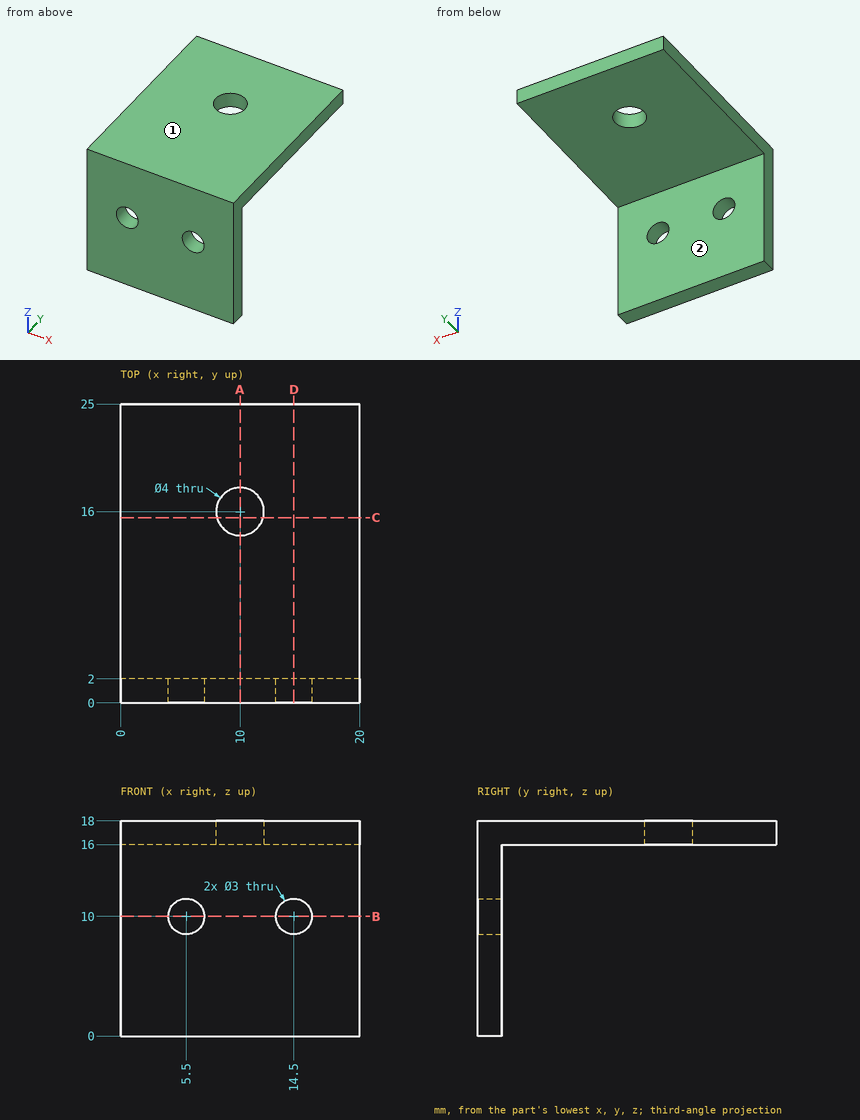
Input: dimensioned drawing with shaded views. Units: mm. Origin: part minimum x, y, z. A direction names the side the tool comes from. Coordinates: 2 decimals unless noted, no trailing zeros. Order: outer loops, then holes, each group sorted by start corner. A loop starts at its lowest first (then second) coordinate and runs counter-clockwise, first axis right, second up. Notation, with made-up numbers: (3, 28) - (59, 28) arc R31 ccw to (59, 54) - close; hole circle Ø4 at (58, 61.25). An arc over 180 degrees is marked (long way). Return JSON: item names as keys, results as strings. Group by question number.
1. Pin query (flat end, axial travel): pin 1 (6 mm diameter, centred on x = 8.5, y = 15.5, fed in from -Z); pin 2 (3.5 mm diameter, centred on x = 14.5, z = 10, fed in from +Y). Return the tip coordinate at first contact, or that it passes through.
2. Material intervals for line 1 along X through (y, z) = (1.1, 10); line 2 along Y through (x, z) = (10, 17.4); line 3 along Z through (x, y) = (14.5, 1.4), sorted ascending. Write a range as [from, to].
3. Cut plane A-A (x = 10). Output: boundary loops of the cut face in (y, z), plus the area to 3 significant figures.
4. Cut plane D-D (x = 14.5). Output: boundary loops of the cut face in (y, z).
5. Cut plane B-B (z = 10). Output: boundary loops of the cut face in (x, y).
6. Cut plane C-C (y = 15.5). Output: boundary loops of the cut face in (x, z), plus the area to 3 significant figures.
7. Set-up query: the marked faces 1 and 2. Return all of +Z, -Z, +X, -X, +Y, -Y with unobstructed straight access to the full face (end or side cutting, diameter ignored); none if empty.
Resolved:
{
 "1": {"pin 1": "stops at z = 16", "pin 2": "stops at y = 2"},
 "2": {"line 1": "x = [0, 4], [7, 13], [16, 20]", "line 2": "y = [0, 14], [18, 25]", "line 3": "z = [0, 8.5], [11.5, 18]"},
 "3": {"outline": "(0, 0) - (2, 0) - (2, 16) - (14, 16) - (14, 18) - (0, 18) - close; (18, 16) - (25, 16) - (25, 18) - (18, 18) - close", "area": "74.0 mm²"},
 "4": {"outline": "(0, 0) - (2, 0) - (2, 8.5) - (0, 8.5) - close; (0, 11.5) - (2, 11.5) - (2, 16) - (25, 16) - (25, 18) - (0, 18) - close"},
 "5": {"outline": "(0, 0) - (4, 0) - (4, 2) - (0, 2) - close; (7, 0) - (13, 0) - (13, 2) - (7, 2) - close; (16, 0) - (20, 0) - (20, 2) - (16, 2) - close"},
 "6": {"outline": "(0, 16) - (8.06, 16) - (8.06, 18) - (0, 18) - close; (11.94, 16) - (20, 16) - (20, 18) - (11.94, 18) - close", "area": "32.3 mm²"},
 "7": {"face 1": "+Z, +X, -X, +Y, -Y", "face 2": "-Z, +X, -X, +Y"}
}
